CAD build for the part. Positions are in the model's coordinates, mm. Give positions to 0.01 mm unless a question says otherwise; leave off trailing zeros. Order: outer loops, then holes, each group sorted by start corner. A loop starts at its lowest first (then second) coordinate and runs counter-clockwise, first axis right, second up.
Item 1: Band-saw the part on D-D on z = -18. Give the cut face in (x, y).
Item 2: Band-saw the part on C-C on z = -75. Give the cut face in (x, y).
Item 3: Wall check: L1, parallel to X at y = 2.95, z = -75; L2, parallel to Z at x = 5, y = 3.75; L3, parallel to X at y = 1.9, z = -44.5. Give the ranges that are in metal, low to high.
Item 4: Flat gauge pin, fed straight in: P1, Ø3, axis at x = 75, z = -150, coming from the +Y side. Where does the tip first touch, or does it go through?
Item 5: Band-saw the part on A-A on z = -122.5. Give the cut face in (x, y).
Item 6: Band-saw the part on B-B on x = 75. Give the cut face in (y, z), plus the area to 3 significant figures.
Item 7: Two-plate mould, pull along Z, no slides. Class faces 1 (the flat face through (39, 0, -81)), 2 (the cylindrical face through (34, 3, -18)), 3 (the flat face through (39, 2, 0)): released by +Z, released by -Z, zero draft, split by the parting line, or undercut.
```python
from build123d import *

# Parameters (mm, degrees)
ESQUISSE1_W              = 80
ESQUISSE1_H              = 160
BOSS_EXTRU_1_DEPTH       = 5
ESQUISSE2_R              = 1.6
ENL_V_MAT_EXTRU_8_DEPTH  = 10
ESQUISSE3_W              = 19.8
ESQUISSE3_H              = 13
ENL_V_MAT_EXTRU_9_DEPTH  = 10
ESQUISSE4_R              = 1.6
ENL_V_MAT_EXTRU_10_DEPTH = 10
ENL_V_MAT_EXTRU_11_DEPTH = 179.955301682
ENL_V_MAT_EXTRU_12_DEPTH = 179.955301682


with BuildPart() as part:
    # Esquisse1 → Boss.-Extru.1 (new body)
    with BuildSketch(Plane(origin=(0, 0, 0), x_dir=(1, 0, 0), z_dir=(0, 1, 0))):
        with Locations((40, 80)):
            Rectangle(ESQUISSE1_W, ESQUISSE1_H)
    extrude(amount=BOSS_EXTRU_1_DEPTH)

    # Esquisse2 → Enlèv. mat.-Extru.8 (cut)
    with BuildSketch(Plane(origin=(0, 0, 0), x_dir=(1, 0, 0), z_dir=(0, 1, 0))):
        with Locations(Location((5, 150, 0), (0, 0, 90))):
            Circle(ESQUISSE2_R)
        with Locations(Location((5, 75, 0), (0, 0, 90))):
            Circle(ESQUISSE2_R)
        with Locations(Location((5, 10, 0), (0, 0, 90))):
            Circle(ESQUISSE2_R)
        with Locations(Location((75, 10, 0), (0, 0, 90))):
            Circle(ESQUISSE2_R)
        with Locations(Location((75, 75, 0), (0, 0, 90))):
            Circle(ESQUISSE2_R)
        with Locations(Location((75, 150, 0), (0, 0, 90))):
            Circle(ESQUISSE2_R)
    extrude(amount=ENL_V_MAT_EXTRU_8_DEPTH, mode=Mode.SUBTRACT)

    # Esquisse3 → Enlèv. mat.-Extru.9 (cut)
    with BuildSketch(Plane(origin=(0, 0, 0), x_dir=(1, 0, 0), z_dir=(0, 1, 0))):
        with Locations((40, 123.5)):
            Rectangle(ESQUISSE3_W, ESQUISSE3_H)
    extrude(amount=ENL_V_MAT_EXTRU_9_DEPTH, mode=Mode.SUBTRACT)

    # Esquisse4 → Enlèv. mat.-Extru.10 (cut)
    with BuildSketch(Plane(origin=(0, 5, 0), x_dir=(1, 0, 0), z_dir=(0, 1, 0))):
        with Locations(Location((31.225, 8, 0), (0, 0, 270))):
            Circle(ESQUISSE4_R)
        with Locations(Location((48.775, 8, 0), (0, 0, 90))):
            Circle(ESQUISSE4_R)
    extrude(amount=-ENL_V_MAT_EXTRU_10_DEPTH, mode=Mode.SUBTRACT)

    # Esquisse5 → Enlèv. mat.-Extru.11 (cut, through all)
    with BuildSketch(Plane(origin=(0, 5, 0), x_dir=(1, 0, 0), z_dir=(0, 1, 0))):
        with BuildLine():
            Line((37.5, 21.5), (42.5, 21.5))
            ThreePointArc((42.5, 21.5), (46, 18), (42.5, 14.5))
            Line((42.5, 14.5), (37.5, 14.5))
            ThreePointArc((37.5, 14.5), (34, 18), (37.5, 21.5))
        make_face()
    extrude(amount=-ENL_V_MAT_EXTRU_11_DEPTH, mode=Mode.SUBTRACT)

    # Esquisse6 → Enlèv. mat.-Extru.12 (cut, through all)
    with BuildSketch(Plane(origin=(0, 5, 0), x_dir=(1, 0, 0), z_dir=(0, 1, 0))):
        with BuildLine():
            Line((30, 50), (50, 50))
            ThreePointArc((50, 50), (55, 45), (50, 40))
            Line((50, 40), (30, 40))
            ThreePointArc((30, 40), (25, 45), (30, 50))
        make_face()
    extrude(amount=-ENL_V_MAT_EXTRU_12_DEPTH, mode=Mode.SUBTRACT)


solid = part.part
```
The answers:
1. outline: (0, 0) - (34, 0) - (34, 5) - (0, 5) - close; (46, 0) - (80, 0) - (80, 5) - (46, 5) - close
2. outline: (0, 0) - (3.4, 0) - (3.4, 5) - (0, 5) - close; (6.6, 0) - (73.4, 0) - (73.4, 5) - (6.6, 5) - close; (76.6, 0) - (80, 0) - (80, 5) - (76.6, 5) - close
3. L1: x = 0 to 3.4, 6.6 to 73.4, 76.6 to 80
3. L2: z = -160 to -151.6, -148.4 to -76.6, -73.4 to -11.6, -8.4 to 0
3. L3: x = 0 to 25.03, 54.97 to 80
4. P1: passes through
5. outline: (0, 0) - (30.1, 0) - (30.1, 5) - (0, 5) - close; (49.9, 0) - (80, 0) - (80, 5) - (49.9, 5) - close
6. outline: (0, -160) - (5, -160) - (5, -151.6) - (0, -151.6) - close; (0, -148.4) - (5, -148.4) - (5, -76.6) - (0, -76.6) - close; (0, -73.4) - (5, -73.4) - (5, -11.6) - (0, -11.6) - close; (0, -8.4) - (5, -8.4) - (5, 0) - (0, 0) - close
6. area: 752 mm2
7. face 1: zero draft
7. face 2: undercut
7. face 3: released by +Z
